Source: CAD feature listing. Evaluate the final solid. Frame: model axes, mm. A direction names the side the tool comes from. Round coordinates to 2 decimals unless told otherwise and drop trailing zeros. Loops run counter-clockwise (first coordinate to the right, second up) from the corner with the lowest first, then second, coordinate; pieces in that order, holes last. Notation, with made-up numbers: (30, 11) - (42, 11) arc R15 cw to (42, 35) - close; hole circle Ø1 at (69, -23). An arc over 180 degrees is marked (long way). One line per question, with ' | ' between items.
from build123d import *

# Parameters (mm, degrees)
SKETCH1_W           = 3.048
SKETCH1_H           = 3.048
BOSS_EXTRUDE1_DEPTH = 4.5593
CAVITY1_START       = 29.845
CAVITY1_OUTLINE_W   = 4.5593
CAVITY1_OUTLINE_H   = 4.5593
CAVITY1_DEPTH       = 95.25
CAVITY1_START_2     = 120.5357
CAVITY1_2_OUTLINE_W = 4.5593
CAVITY1_2_OUTLINE_H = 19.05
CAVITY1_2_DEPTH     = 4.5593


# Read off the part's stored shape, not the designer's step: Cavity1
with BuildPart() as part:
    # Sketch1 → Boss-Extrude1 (new body)
    with BuildSketch(Plane(origin=(0, 0, 0), x_dir=(1, 0, 0), z_dir=(0, 1, 0))):
        Polygon((125.095, -23.6093), (-125.095, -23.6093), (-125.095, -1.524), (-122.047, -1.524), (-122.047, 1.524), (-125.095, 1.524), (-125.095, 23.6093), (125.095, 23.6093), align=None)
        with Locations((-99.695, 0)):
            Rectangle(SKETCH1_W, SKETCH1_H, mode=Mode.SUBTRACT)
    extrude(amount=BOSS_EXTRUDE1_DEPTH)

    # Cavity1 outline → Cavity1 (cut)
    with BuildSketch(Plane.YZ.offset(CAVITY1_START)):
        with Locations((2.27965, 21.32965)):
            Rectangle(CAVITY1_OUTLINE_W, CAVITY1_OUTLINE_H)
        with Locations((2.27965, -21.32965)):
            Rectangle(CAVITY1_OUTLINE_W, CAVITY1_OUTLINE_H)
    extrude(amount=CAVITY1_DEPTH, mode=Mode.SUBTRACT)

    # Cavity1 2 outline → Cavity1 2 (cut)
    with BuildSketch(Plane.YZ.offset(CAVITY1_START_2)):
        with Locations((2.27965, -9.525)):
            Rectangle(CAVITY1_2_OUTLINE_W, CAVITY1_2_OUTLINE_H)
    extrude(amount=CAVITY1_2_DEPTH, mode=Mode.SUBTRACT)


solid = part.part
1. Contact query for flat-ended pins moving along their axis: P1, Ø10, axis at x = 33.5, z = -7, coming from the -Y side; P2, Ø1.4, axis at x = 75, y = 3, coming from the +Z side; P3, Ø1.4, axis at y = 2.5, z = -20.5, coming from the +X side (3 decimals); P4, Ø1.5, axis at x = 93.5, y = 4, coming from the -Z side. Output: stop coordinate, or through.
Worked out:
P1: stops at y = 0 | P2: stops at z = 19.05 | P3: stops at x = 29.845 | P4: stops at z = -19.05
2. Access query for faces 1 (the flat face through (-125.095, 2, 13)), 2 (the flat face through (77, 2, 19.05)), 3 (the flat face through (75, 2, -19.05)). Directions: +Z, -Z, +X, -X, +Y, -Y. A direction counts if a zero-diameter tool reaches every point of the face in a straight line with its end or side. Return the directions, or none.
Worked out:
face 1: +Z, -Z, -X, +Y, -Y | face 2: +Z, +X, +Y, -Y | face 3: -Z, +X, +Y, -Y
3. Section query C-C, the plane z = -14.5. Return loops of the section in (x, y) (3 decimals).
Worked out:
outline: (-125.095, 0) - (120.536, 0) - (120.536, 4.559) - (-125.095, 4.559) - close
4. Section query A-A, the plane y = 1.65. Return loops of the section in (x, z) (3 decimals).
Worked out:
outline: (-125.095, -23.609) - (29.845, -23.609) - (29.845, -19.05) - (120.536, -19.05) - (120.536, 0) - (125.095, 0) - (125.095, 19.05) - (29.845, 19.05) - (29.845, 23.609) - (-125.095, 23.609) - (-125.095, 1.524) - (-122.047, 1.524) - (-122.047, -1.524) - (-125.095, -1.524) - close; hole (-101.219, -1.524) - (-98.171, -1.524) - (-98.171, 1.524) - (-101.219, 1.524) - close
5. Material intervals for probe 1 along Z at (x, y) = (84.5, 1.15); probe 2 along X at (y, z) = (1.6, -15) (3 decimals); probe 3 along X at (y, z) = (0.3, 22.5) (3 decimals), sorted ascending.
Worked out:
probe 1: z = -19.05 to 19.05 | probe 2: x = -125.095 to 120.536 | probe 3: x = -125.095 to 29.845
6. Section query B-B, the plane x = 57. Return loops of the section in (y, z), plus the area to 3 significant figures.
Worked out:
outline: (0, -19.05) - (4.56, -19.05) - (4.56, 19.05) - (0, 19.05) - close | area: 174 mm2
